Geometry: final body of the model. Coordinates: model frame, mm. Give positions to 0.01 mm unless a question says otherwise; leave off trailing zeros. Write each loop counter-clockwise with the first axis right and the second up, starting at its lowest first coordinate (ties: lowest second). Pieces come first, ordered by that corner, then holes.
from build123d import *

# Parameters (mm, degrees)
CUT_EXTRUDE1_DEPTH = 0.9


with BuildPart() as part:
    # Sketch1 → Revolve1 (revolve)
    with BuildSketch(Plane.XY):
        with BuildLine():
            Line((0, 0), (0, 0.742857779))
            ThreePointArc((0, 0.742857779), (0.360668212, 1.718523233), (1.269230769, 2.225))
            ThreePointArc((1.269230769, 2.225), (1.430088727, 2.179291942), (1.5, 2.027381037))
            Line((1.5, 2.027381037), (1.5, 1.4))
            ThreePointArc((1.5, 1.4), (1.558578644, 1.258578644), (1.7, 1.2))
            Line((1.7, 1.2), (5.65, 1.2))
            Line((5.65, 1.2), (6, 0.85))
            Line((6, 0.85), (6, 0))
            Line((6, 0), (0, 0))
        make_face()
    revolve(axis=Axis((0, 0, 0), (-1, 0, 0)))

    # Sketch2 → Cut-Extrude1 (cut)
    with BuildSketch(Plane.ZY):
        Polygon((0.75, -0.433012702), (0.75, 0.433012702), (0, 0.866025404), (-0.75, 0.433012702), (-0.75, -0.433012702), (0, -0.866025404), align=None)
    extrude(amount=-CUT_EXTRUDE1_DEPTH, mode=Mode.SUBTRACT)


solid = part.part
Q1. Pin query (flat end, axial travel): P1, Ø2, axis at x = 3, y = -0.5, coming from the +Z side; P2, Ø1.7, axis at y = 0, z = -0.5, coming from the -X side; P3, Ø1, axis at x = 0.5, y = 0, coming from the -Z side. Return the tip coordinate at first contact, or that it passes through.
Filled sheet:
P1: stops at z = 1.2
P2: stops at x = 0
P3: stops at z = -2.16
Q2. Section A-A on x = 4.75. Output: boundary loops of the cut face in (y, z).
Filled sheet:
outline: circle Ø2.4 at (0, 0)
Q3. Ray query, line 1 along Y through (x, z) = (4.1, 0); line 2 along X through (y, z) = (-0.1, -0.3); line 3 along X through (y, z) = (-1.4, 0.2). Return the intervals inside material, ascending.
Filled sheet:
line 1: y = -1.2 to 1.2
line 2: x = 0.9 to 6
line 3: x = 0.16 to 1.5
Q4. Pull-direction query (Y, two-part tool) for faces 1 (the flat face through (0.4, 0, -0.75)), 2 (the cylindrical face through (3.7, 0.65, -1.01)), 3 (the flat face through (6, 0, 0)); classes: released by +Y, released by -Y, zero draft, split by the parting line, or undercut.
Filled sheet:
face 1: undercut
face 2: split by the parting line
face 3: zero draft
Q5. Section B-B on x = 1.35. Output: boundary loops of the cut face in (y, z), plus the area to 3 significant figures.
Filled sheet:
outline: circle Ø4.44 at (0, 0)
area: 15.5 mm2
